Build history of the part. All positions in model axes, mm. Round coordinates to 2 decimals unless told otherwise and drop trailing zeros. Write each loop counter-clockwise with the first axis right and the second up, starting at its lowest first coordinate (ties: lowest second). Pieces come first, ordered by that corner, then holes.
from build123d import *

# Parameters (mm, degrees)
PAD_DEPTH = 0.8
FILLET_R  = 0.2


with BuildPart() as part:
    # Sketch → Pad (new body)
    with BuildSketch(Plane.XY):
        with BuildLine():
            Line((0.3, 0), (19.7, 0))
            ThreePointArc((19.7, 0), (19.912132, 0.087868), (20, 0.3))
            Line((20, 16.3), (20, 0.3))
            ThreePointArc((20, 16.3), (19.912132, 16.512132), (19.7, 16.6))
            Line((19.7, 16.6), (0.3, 16.6))
            ThreePointArc((0.3, 16.6), (0.087868, 16.512132), (0, 16.3))
            Line((0, 16.3), (0, 0.3))
            ThreePointArc((0, 0.3), (0.087868, 0.087868), (0.3, 0))
        make_face()
        with BuildLine():
            Line((19, 15.8), (19, 0.8))
            Line((19, 0.8), (1, 0.8))
            Line((1, 0.8), (1, 11.428862))
            ThreePointArc((1.046791, 11.55742), (1.012061, 11.497266), (1, 11.428862))
            Line((1.046791, 11.55742), (4.546791, 15.728558))
            ThreePointArc((4.7, 15.8), (4.615476, 15.781262), (4.546791, 15.728558))
            Line((4.7, 15.8), (19, 15.8))
        make_face(mode=Mode.SUBTRACT)
    extrude(amount=PAD_DEPTH)

    # Fillet
    fillet_edges = [part.edges().sort_by_distance(p)[0] for p in [
        (0, 8.3, 0.8),
        (0, 8.3, 0),
        (1, 6.114431, 0),
        (19, 8.3, 0),
        (10, 0.8, 0),
        (11.85, 15.8, 0),
        (2.796791, 13.642989, 0),
        (2.796791, 13.642989, 0.8),
        (1, 6.114431, 0.8),
        (11.85, 15.8, 0.8),
        (19, 8.3, 0.8),
        (10, 0.8, 0.8),
    ]]
    fillet(fillet_edges, radius=FILLET_R)


solid = part.part
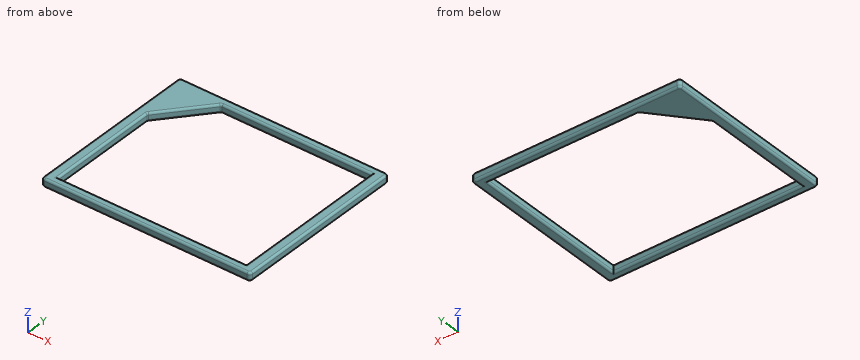
1) Slice it at B-B (x = 8.25). Write the cut outline in (y, z), plus the area to 3 significant figures.
Results:
outline: (0, 0.2) arc R0.2 ccw to (0.2, 0) - (0.6, 0) arc R0.2 ccw to (0.8, 0.2) - (0.8, 0.6) arc R0.2 ccw to (0.6, 0.8) - (0.2, 0.8) arc R0.2 ccw to (0, 0.6) - close; (15.8, 0.2) arc R0.2 ccw to (16, 0) - (16.4, 0) arc R0.2 ccw to (16.6, 0.2) - (16.6, 0.6) arc R0.2 ccw to (16.4, 0.8) - (16, 0.8) arc R0.2 ccw to (15.8, 0.6) - close
area: 1.21 mm2
2) Wall check: L1, parallel to X at y = 5.75, z = 0.25; L2, parallel to Y at x = 17, z = 0.2; L3, parallel to Y at x = 2.25, z = 0.1. Give the ranges that are in metal, low to high.
Results:
L1: x = 0 to 1, 19 to 20
L2: y = 0 to 0.8, 15.8 to 16.6
L3: y = 0.03 to 0.77, 13.03 to 16.57
3) Slice it at A-A (y = 1.25). Write the cut outline in (x, z), plus the area to 3 significant figures.
Results:
outline: (0, 0.2) arc R0.2 ccw to (0.2, 0) - (0.8, 0) arc R0.2 ccw to (1, 0.2) - (1, 0.6) arc R0.2 ccw to (0.8, 0.8) - (0.2, 0.8) arc R0.2 ccw to (0, 0.6) - close; (19, 0.2) arc R0.2 ccw to (19.2, 0) - (19.8, 0) arc R0.2 ccw to (20, 0.2) - (20, 0.6) arc R0.2 ccw to (19.8, 0.8) - (19.2, 0.8) arc R0.2 ccw to (19, 0.6) - close
area: 1.53 mm2
